Can you work these out from the model? Positions are in its coordinate system, mm. Round coordinates to 2 decimals unless told otherwise and drop trailing zeros. Write each loop counter-clockwise with the first axis right and the second up, starting at its lowest first coordinate (ties: lowest second). Pieces come first, ordered by that corner, then holes.
Q1. If we section it at A-A (y = 98): Please give me the cut outline in (x, z).
Q2. If we section it at C-C (z = 65): Please give me the cut outline in (x, y), plus the area to 3 significant figures.
Q3. Please list where these lines run through material, in increasing order: line 1 along Z through (x, y) = (-0.5, 45); line 2 along Z through (x, y) = (14.5, -3.5); line 3 along X through (y, z) = (57.5, -13).
Q4. If we section it at B-B (x = -59): Please give me the cut outline in (y, z).
Q5. I'm going to push flat-ended pins straight in: pin 1 Ø1 at (x, y) = (24, 11) entering from -Z; pin 2 Ø4 at (x, y) = (53.5, -19) entering from +Z; pin 3 Ø6 at (y, z) = (-35.5, -18.5) entering from +X. Where does each tip first touch, or does it pass through?
from build123d import *

# Parameters (mm, degrees)
F0_R     = 75.5472350888
F1_DEPTH = 127
F4_DEPTH = 6.35


with BuildPart() as f1:
    # F0 (on Front) → F1 (new body, symmetric)
    with BuildSketch(Plane.XZ):
        Circle(F0_R)
    extrude(amount=F1_DEPTH, both=True)

    # F3 (on offset) → F4 (join, symmetric)
    with BuildSketch(Plane.XY.offset(75.184)):
        with BuildLine():
            add(Edge.make_bspline(
                [(0, -26.8084928393), (27.3186761033, -26.8084928393), (13.6593380516, 13.4042464197), (0, 53.6169856787), (-13.6593380516, 13.4042464197), (-27.3186761033, -26.8084928393), (0, -26.8084928393)],
                knots=[0, 0, 0, 2.0943951024, 2.0943951024, 4.1887902048, 4.1887902048, 6.2831853072, 6.2831853072, 6.2831853072], degree=2, weights=[1, 0.5, 1, 0.5, 1, 0.5, 1]))
        make_face()
    extrude(amount=F4_DEPTH, both=True)


solid = f1.part
A:
1. outline: circle Ø151.09 at (0, 0)
2. outline: (-38.5, -127) - (38.5, -127) - (38.5, 127) - (-38.5, 127) - close
2. area: 19,600 mm2
3. line 1: z = -75.55 to 75.55
3. line 2: z = -74.14 to 81.53
3. line 3: x = -74.42 to 74.42
4. outline: (-127, -47.18) - (127, -47.18) - (127, 47.18) - (-127, 47.18) - close
5. pin 1: stops at z = -71.8
5. pin 2: stops at z = 55.27
5. pin 3: stops at x = 73.94
